Part print with two shaded views. Sizes in mm from the minimum x, y, z corner. Give positions to 0.01 mm unless a question says otherwise; leave off trailing zeros. Write each loop counter-clockwise with the first axis right and the second up, starting at its lowest first coordinate (ties: lowest second). Pieces come first, ordered by that corner, then holes. Notation, with made-up numbers: (41.25, 65.5) - (77.25, 65.5) arc R16 cw to (77.25, 69.5) - close; hole circle Ø4 at (35.5, 17.25). An arc over 180 degrees is marked (long way). One line per item, written item: value. Start each with the question number.
(1) Probe L1, parallel to Y at x = 32, z = 1.7; L2, parallel to Y at x = 3, z = 1.25; L3, parallel to Y at x = 37.5, z = 2.95. List the from-to ranges inside material, lowest first.
(2) Cut at A-A, the plane x = 32. List the corners of the cut face in (y, z).
(3) Cut at C-C, the plane z = 2.55. List the corners of the cut face in (x, y), and give its area (3 significant figures).
(4) Drop a flat-ended pin along its axis: P1, Ø2.5, axis at x = 32, y = 8, coming from the +Z side. Give the stop position or say it passes through.
(5) Cut at B-B, the plane y = 8. List the corners of the cut face in (x, z), and give its area (3 significant figures).
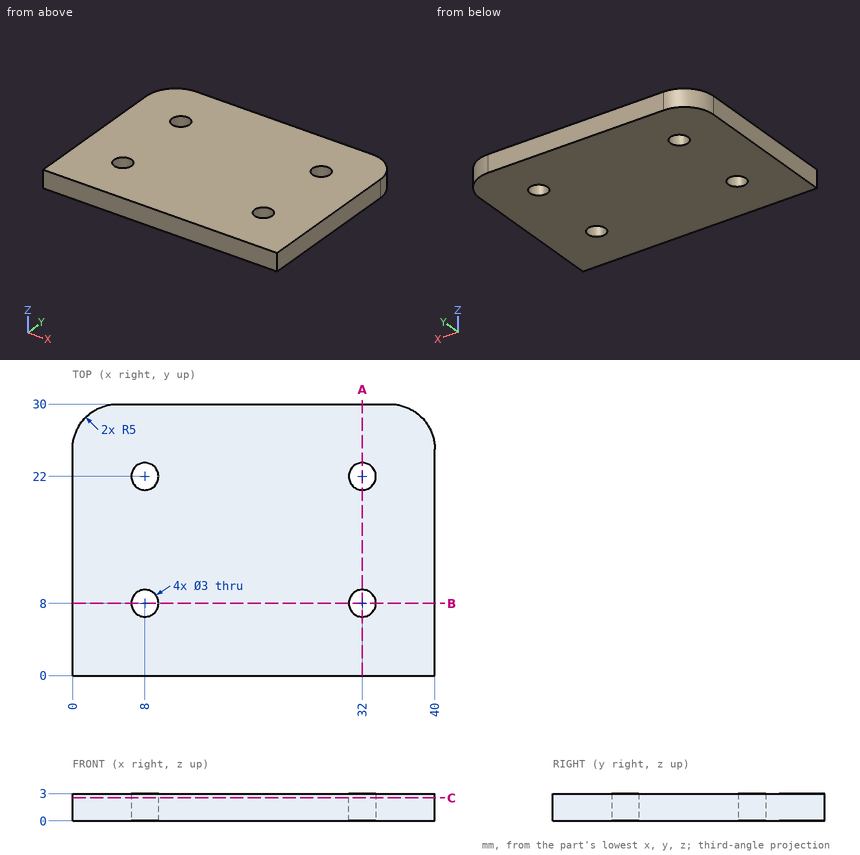
Answers follow:
1. L1: y = 0 to 6.5, 9.5 to 20.5, 23.5 to 30
1. L2: y = 0 to 29.58
1. L3: y = 0 to 29.33
2. outline: (0, 0) - (6.5, 0) - (6.5, 3) - (0, 3) - close; (9.5, 0) - (20.5, 0) - (20.5, 3) - (9.5, 3) - close; (23.5, 0) - (30, 0) - (30, 3) - (23.5, 3) - close
3. outline: (0, 0) - (40, 0) - (40, 25) arc R5 ccw to (35, 30) - (5, 30) arc R5 ccw to (0, 25) - close; hole circle Ø3 at (8, 8); hole circle Ø3 at (8, 22); hole circle Ø3 at (32, 8); hole circle Ø3 at (32, 22)
3. area: 1,160 mm²
4. P1: passes through
5. outline: (0, 0) - (6.5, 0) - (6.5, 3) - (0, 3) - close; (9.5, 0) - (30.5, 0) - (30.5, 3) - (9.5, 3) - close; (33.5, 0) - (40, 0) - (40, 3) - (33.5, 3) - close
5. area: 102 mm²
